from build123d import *

# Parameters (mm, degrees)
SKETCH_W            = 220
SKETCH_H            = 220
PAD_DEPTH           = 5
PAD001_DEPTH        = 220
LINEARPATTERN_COUNT = 2
LINEARPATTERN_PITCH = 210
SKETCH003_W         = 10
SKETCH003_H         = 200
PAD003_DEPTH        = 10


with BuildPart() as part:
    # Sketch → Pad (new body)
    with BuildSketch(Plane.XY):
        Rectangle(SKETCH_W, SKETCH_H)
    extrude(amount=PAD_DEPTH)

    # Sketch001 (on Face2 of Pad) → Pad001 (join)
    with BuildSketch(Plane.YZ.offset(110)):
        Polygon((-110, 5), (-110, 65), (-113, 65), (-113, 75), (-97, 75), (-97, 65), (-100, 65), (-100, 5), align=None)
    pad001 = extrude(amount=-PAD001_DEPTH)

    # LinearPattern: Pad001 ×2
    with Locations(*[(0, i * LINEARPATTERN_PITCH, 0) for i in range(1, LINEARPATTERN_COUNT)]):
        add(pad001)

    # Sketch003 (on Face7 of LinearPattern) → Pad003 (join)
    with BuildSketch(Plane.XY.offset(5)):
        with Locations((-65, 0)):
            Rectangle(SKETCH003_W, SKETCH003_H)
        with Locations((65, 0)):
            Rectangle(SKETCH003_W, SKETCH003_H)
    extrude(amount=PAD003_DEPTH)


solid = part.part
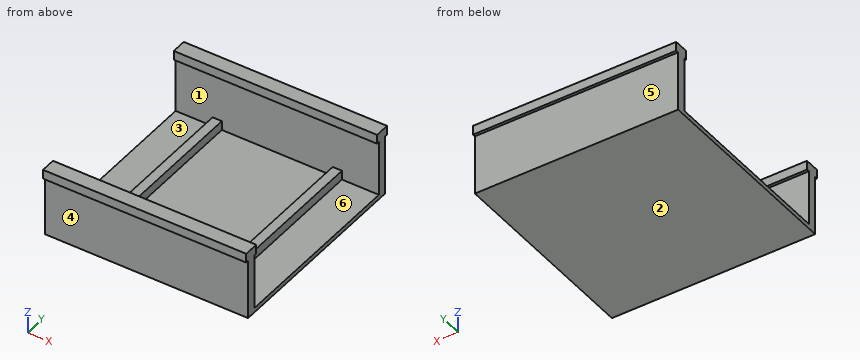
Source: CAD feature listing. Evaluate the final solid. Frame: model axes, mm. Face numbers are marked on the shaded views. A direction names the side the tool comes from. Round coordinates to 2 decimals unless told otherwise and drop trailing zeros. Loops run counter-clockwise (first coordinate to the right, second up) from the corner with the lowest first, then second, coordinate; pieces in that order, holes last. Notation, with made-up numbers: (26.5, 58) - (57.5, 58) arc R14 cw to (57.5, 62) - close; hole circle Ø6 at (78, 76.5). An arc over 180 degrees is marked (long way). Write item = value, one per line. Start each with the question number.
Item 1: Reachability of the marked faces 1 and 2 from +Z, -Z, +X, -X, +Y, -Y: full face, straight path, thin tool, end or side. Return the list, or none.
Item 2: Section query A-A on z = 39. Output: boundary loops of the cut face in (x, y), plus the area to 3 significant figures.
Item 3: Section query C-C on y = -4. Output: boundary loops of the cut face in (x, z), plus the area to 3 significant figures.
Item 4: Section query B-B on x = 31.5. Output: boundary loops of the cut face in (y, z), plus the area to 3 significant figures.
Item 5: First-contact query: pin 1 Ø3.5 at (x, y) = (3, -98.5) entering from -Z; pin 2 Ø12 at (x, z) = (81, 38.5) entering from -Y; pin 3 Ø3.5 at (x, y) = (-12, 112) entering from -Z; pin 4 Ø6 at (y, z) = (-27.5, 13) entering from +X. Flat tips, straight axial feed; report the tip coordinate or a pass-through.
Item 6: Material intervals for line 1 (X direction, y = -92, z = 10); line 2 (Y direction, x = -45, z = 52.5); line 3 (Z direction, x = 18.5, y = 79), sorted ascending.
Item 7: Mould query, pull axis Y, two halves, no side actions, for the marked faces 3, 4, 5 and 6. Classes: released by +Y, released by -Y, zero draft, split by the parting line, or undercut.
Results list:
q1.face_1 = none
q1.face_2 = -Z, +X, -X, +Y, -Y
q2.outline = (-110, -110) - (110, -110) - (110, -100) - (-110, -100) - close; (-110, 100) - (110, 100) - (110, 110) - (-110, 110) - close
q2.area = 4,400 mm²
q3.outline = (-110, 0) - (110, 0) - (110, 5) - (70, 5) - (70, 15) - (60, 15) - (60, 5) - (-60, 5) - (-60, 15) - (-70, 15) - (-70, 5) - (-110, 5) - close
q3.area = 1,300 mm²
q4.outline = (-113, 65) - (-110, 65) - (-110, 0) - (110, 0) - (110, 65) - (113, 65) - (113, 75) - (97, 75) - (97, 65) - (100, 65) - (100, 5) - (-100, 5) - (-100, 65) - (-97, 65) - (-97, 75) - (-113, 75) - close
q4.area = 2,620 mm²
q5.pin_1 = 0
q5.pin_2 = -110
q5.pin_3 = 65
q5.pin_4 = 70
q6.line_1 = -70 to -60, 60 to 70
q6.line_2 = -110 to -100, 100 to 110
q6.line_3 = 0 to 5
q7.face_3 = undercut
q7.face_4 = released by -Y
q7.face_5 = released by +Y
q7.face_6 = undercut
